Can you work these out from the model? Positions are in its coordinate system, mm. A direction names the side the tool comes from. Coordinates: 2 decimals unless noted, no trailing zeros. Order: outer loops, then holes, each group sorted by start corner. A loop starts at its lowest first (then second) coordinate and runs counter-clockwise, first axis right, second up. Notation, with made-up numbers: (-2, -34) -> (28, -34) arc R26 cw to (28, -2) -> close; hole circle Ø9 at (19, -23). An arc over 180 degrees is marked (long way). Answer in a Markdown table with one row per item.
```python
from build123d import *

# Parameters (mm, degrees)
BOSS_EXTRUDE1_DEPTH = 10
SKETCH2_R           = 3
BOSS_EXTRUDE2_DEPTH = 5
SKETCH3_R           = 1.778
CUT_EXTRUDE1_DEPTH  = 5


with BuildPart() as part:
    # Sketch1 → Boss-Extrude1 (new body)
    with BuildSketch(Plane(origin=(0, 0, 0), x_dir=(1, 0, 0), z_dir=(0, 1, 0))):
        with BuildLine():
            Line((-5.780656579, 24.018987342), (4.219343421, 24.018987342))
            ThreePointArc((4.219343421, 24.018987342), (7.754877327, 22.554521248), (9.219343421, 19.018987342))
            Line((9.219343421, 19.018987342), (9.219343421, 14.018987342))
            Line((9.219343421, 14.018987342), (19.219343421, 14.018987342))
            Line((19.219343421, 14.018987342), (0, -35.981012658))
            Line((0, -35.981012658), (-20.780656579, 14.018987342))
            Line((-20.780656579, 14.018987342), (-10.780656579, 14.018987342))
            Line((-10.780656579, 14.018987342), (-10.780656579, 19.018987342))
            ThreePointArc((-10.780656579, 19.018987342), (-9.316190485, 22.554521248), (-5.780656579, 24.018987342))
        make_face()
    extrude(amount=BOSS_EXTRUDE1_DEPTH)

    # Sketch2 → Boss-Extrude2 (add)
    with BuildSketch(Plane.XZ):
        with Locations((0.635595912, -21.018987342)):
            Circle(SKETCH2_R)
    extrude(amount=BOSS_EXTRUDE2_DEPTH)

    # Sketch3 → Cut-Extrude1 (cut)
    with BuildSketch(Plane.XZ.offset(5)):
        with Locations((0.635595912, -21.018987342)):
            Circle(SKETCH3_R)
    extrude(amount=-CUT_EXTRUDE1_DEPTH, mode=Mode.SUBTRACT)


solid = part.part
```
(1) We'd pull the mould along Z, two halves only. Please class faces 4 (the flat face through (1, 0, -21)), 5 (the flat face through (3, -5, -21)), 6 (the flat face through (14, 5, -14.019)), 7 (the cylindrical face through (0.25, -2.535, -22.755)): +Z half, -Z half, draft (parallel to the pull), parting line (faces both ways), or undercut.
Response values:
| item | result |
|---|---|
| face 4 | undercut |
| face 5 | draft |
| face 6 | -Z half |
| face 7 | undercut |
(2) Suppose I cut it at B-B (z = -15.5). Please give me the cut outline in (x, y), and give its area (3 significant figures).
Response values:
| item | result |
|---|---|
| outline | (-10.78, 0) -> (9.22, 0) -> (9.22, 10) -> (-10.78, 10) -> close |
| area | 200 mm2 |
(3) Suppose I cut it at C-C (x = 16). Please give me the cut outline in (y, z), and give its area (3 significant figures).
Response values:
| item | result |
|---|---|
| outline | (0, -14.02) -> (10, -14.02) -> (10, -5.64) -> (0, -5.64) -> close |
| area | 83.8 mm2 |
(4) Will these pins go through, and if not, where does the flat tip stop? pin 1 Ø2 at (x, y) = (-10, 1) entering from -Z; pin 2 Ø1.5 at (y, z) = (1, -8) entering from -X; pin 3 Ø5.5 at (y, z) = (3.5, -15.5) entering from -X; pin 4 Ø1.5 at (x, y) = (12.5, -1.5) entering from -Z.
Response values:
| item | result |
|---|---|
| pin 1 | z = -22.84 |
| pin 2 | x = -18.59 |
| pin 3 | x = -20.78 |
| pin 4 | through |
(5) Suppose I cut it at D-D (y = -2.25). Please give me the cut outline in (x, z), and give its area (3 significant figures).
Response values:
| item | result |
|---|---|
| outline | circle Ø6 at (0.64, -21.02); hole circle Ø3.56 at (0.64, -21.02) |
| area | 18.3 mm2 |
(6) I need wall thicknesses on line 1 (Y direction, x = -18.5, z = -11); line 2 (Z direction, x = -4, y = 0.25); line 3 (X direction, y = 5.25, z = 4.5). Which ranges of each line are inside material? Lowest first, please. Write a range as [from, to].
Response values:
| item | result |
|---|---|
| line 1 | [0, 10] |
| line 2 | [-24.02, 26.36] |
| line 3 | [-13.08, 12.1] |
(7) Suppose I cut it at A-A (y = 6.5). Please give me the cut outline in (x, z).
Response values:
| item | result |
|---|---|
| outline | (-20.78, -14.02) -> (-10.78, -14.02) -> (-10.78, -19.02) arc R5 ccw to (-5.78, -24.02) -> (4.22, -24.02) arc R5 ccw to (9.22, -19.02) -> (9.22, -14.02) -> (19.22, -14.02) -> (0, 35.98) -> close |
(8) On a 3-axis mill with a long thin cutter (end or side, diameter ignored), from which of +Z, -Z, +X, -X, +Y, -Y can I reach the whole of each face in a straight line? I mean faces 1 (the cylindrical face through (2.25, -2.46, -18.49)), 2 (the flat face through (9.219, 5, -17)), 3 (the flat face through (-16, 5, -14.019)). Say none if no direction works.
Response values:
| item | result |
|---|---|
| face 1 | -Y |
| face 2 | -Z, +X, +Y, -Y |
| face 3 | -Z, -X, +Y, -Y |
